```python
from build123d import *

# Parameters (mm, degrees)
SKETCH_W     = 14
SKETCH_H     = 15
PAD_DEPTH    = 3
SKETCH001_W  = 2.5
SKETCH001_H  = 12.5
PAD001_DEPTH = 10
SKETCH002_W  = 6.75
SKETCH002_H  = 6.75
PAD002_DEPTH = 5


with BuildPart() as part:
    # Sketch → Pad (new body)
    with BuildSketch(Plane.XY):
        with Locations((7, 7.5)):
            Rectangle(SKETCH_W, SKETCH_H)
    extrude(amount=PAD_DEPTH)

    # Sketch001 (on Face6 of Pad) → Pad001 (join)
    with BuildSketch(Plane.XY.offset(3)):
        with Locations((11.5, 7.5)):
            Rectangle(SKETCH001_W, SKETCH001_H)
    extrude(amount=PAD001_DEPTH)

    # Sketch002 (on Face5 of Pad001) → Pad002 (join)
    with BuildSketch(Plane.XY.offset(3)):
        with Locations((4.875, 4.625)):
            Rectangle(SKETCH002_W, SKETCH002_H)
    extrude(amount=PAD002_DEPTH)


solid = part.part
```
Verification items for the finished model (mm, model axes). A direction names the side the tool comes from. Round coordinates to 2 decimals unless told otherwise and drop trailing zeros. Write each loop counter-clockwise with the first axis right and the second up, starting at its lowest first coordinate (ties: lowest second). Pieces come first, ordered by that corner, then holes.
1. Scan lines: L1, parallel to X at y = 3, z = 7.75; L2, parallel to Z at x = 5.5, y = 1; L3, parallel to Z at x = 6.5, y = 2. Record each from-to range of solid material in increasing order.
2. Draft check along X on faces 5 (the flat face through (0, 7, 1)), 6 (the flat face through (7, 8, 0)), 7 (the flat face through (8.25, 5, 5)). Enter one of: +X half, -X half, draft (parallel to the pull), parting line (faces both ways), or undercut.
3. Access from +Z, -Z, +X, -X, +Y, -Y to the whole of each face (thin tool, end or side, straight path). Record for faces 1 (the flat face through (11, 13.75, 8)), 2 (the flat face through (1.5, 5, 5)), 3 (the flat face through (5, 8, 5)), 4 (the flat face through (5, 1.25, 5)).
4. Gauge pin test, flat ends, axial feed: P1, Ø1.5, axis at x = 7.5, z = 4.5, coming from the -Y side; P2, Ø5.5, axis at x = 4, y = 4, coming from the +Z side; P3, Ø1.5, axis at y = 4.5, z = 5, coming from the -X side. Record the tip position at first contact, or that the pin passes through.
5. Section check A-A on z = 7.75. Enter the section's corners in (x, y).
6. Section check B-B on x = 7.5. Enter the section's corners in (y, z), plus the area to 4 significant figures.
7. Section check C-C on y = 4.5. Enter the section's corners in (x, z), plus the area to 3 significant figures.
8. Section check D-D on x = 11.75. Enter the section's corners in (y, z).
Answer:
1. L1: x = 1.5 to 8.25, 10.25 to 12.75
1. L2: z = 0 to 3
1. L3: z = 0 to 8
2. face 5: -X half
2. face 6: draft
2. face 7: undercut
3. face 1: +Z, +X, -X, +Y
3. face 2: +Z, -X, +Y, -Y
3. face 3: +Z, -X, +Y
3. face 4: +Z, +X, -X, -Y
4. P1: stops at y = 1.25
4. P2: stops at z = 8
4. P3: stops at x = 1.5
5. outline: (1.5, 1.25) - (8.25, 1.25) - (8.25, 8) - (1.5, 8) - close; (10.25, 1.25) - (12.75, 1.25) - (12.75, 13.75) - (10.25, 13.75) - close
6. outline: (0, 0) - (15, 0) - (15, 3) - (8, 3) - (8, 8) - (1.25, 8) - (1.25, 3) - (0, 3) - close
6. area: 78.75 mm2
7. outline: (0, 0) - (14, 0) - (14, 3) - (12.75, 3) - (12.75, 13) - (10.25, 13) - (10.25, 3) - (8.25, 3) - (8.25, 8) - (1.5, 8) - (1.5, 3) - (0, 3) - close
7. area: 101 mm2
8. outline: (0, 0) - (15, 0) - (15, 3) - (13.75, 3) - (13.75, 13) - (1.25, 13) - (1.25, 3) - (0, 3) - close
